from build123d import *

# Parameters (mm, degrees)
SKETCH_1_R          = 21.75
SKETCH_1_R_2        = 14.75
EXTRUDE_1_DEPTH     = 55
CUT_EXTRUDE_START   = -5
SKETCH_2_R          = 18.75
SKETCH_2_R_2        = 14.75
CUT_EXTRUDE_1_DEPTH = 59.016862823
SKETCH_3_R          = 1.25
CUT_EXTRUDE_2_DEPTH = 5


with BuildPart() as part:
    # ｽｹｯﾁ1 → ﾎﾞｽ - 押し出し1 (new body)
    with BuildSketch(Plane(origin=(0, 0, 0), x_dir=(1, 0, 0), z_dir=(0, 1, 0))):
        with Locations(Location((0, 0, 0), (0, 0, 270))):
            Circle(SKETCH_1_R)
        with Locations(Location((0, 0, 0), (0, 0, 270))):
            Circle(SKETCH_1_R_2, mode=Mode.SUBTRACT)
    extrude(amount=EXTRUDE_1_DEPTH)

    # ｽｹｯﾁ2 → ｶｯﾄ - 押し出し1 (cut, through all)
    with BuildSketch(Plane(origin=(0, 55, 0), x_dir=(1, 0, 0), z_dir=(0, 1, 0)).offset(CUT_EXTRUDE_START)):
        with Locations(Location((0, 0, 0), (0, 0, 270))):
            Circle(SKETCH_2_R)
        with Locations(Location((0, 0, 0), (0, 0, 270))):
            Circle(SKETCH_2_R_2, mode=Mode.SUBTRACT)
    extrude(amount=-CUT_EXTRUDE_1_DEPTH, mode=Mode.SUBTRACT)

    # ｽｹｯﾁ3 → ｶｯﾄ - 押し出し2 (cut)
    with BuildSketch(Plane(origin=(0, 55, 0), x_dir=(1, 0, 0), z_dir=(0, 1, 0))):
        with Locations(Location((0, 18.25, 0), (0, 0, 270))):
            Circle(SKETCH_3_R)
        with Locations(Location((18.25, 0, 0), (0, 0, 270))):
            Circle(SKETCH_3_R)
        with Locations(Location((0, -18.25, 0), (0, 0, 270))):
            Circle(SKETCH_3_R)
        with Locations(Location((-18.25, 0, 0), (0, 0, 270))):
            Circle(SKETCH_3_R)
    extrude(amount=-CUT_EXTRUDE_2_DEPTH, mode=Mode.SUBTRACT)


solid = part.part
Geometry check sheet. Reference: the model listing, model coordinates, mm. A direction names the side the tool comes from. Give positions to 0.01 mm unless a question says otherwise; leave off trailing zeros. Order: outer loops, then holes, each group sorted by start corner. A loop starts at its lowest first (then second) coordinate and runs counter-clockwise, first axis right, second up.
1) Cross-section at C-C (x = 10). Record the boundary of the cut face in (y, z), then the cut area to 3 significant figures.
Results are:
outline: (0, -19.31) - (55, -19.31) - (55, -10.84) - (50, -10.84) - (50, -15.86) - (0, -15.86) - close; (0, 15.86) - (50, 15.86) - (50, 10.84) - (55, 10.84) - (55, 19.31) - (0, 19.31) - close
area: 430 mm2
2) Gauge pin test, flat ends, axial feed: pin 1 (10 mm diameter, centred on x = -2.5, y = 13, fed in from +Z); pin 2 (2 mm diameter, centred on x = 0, z = -18.25, fed in from +Y); pin 3 (3 mm diameter, centred on x = -15, y = 7.5, fed in from -Z); pin 4 (2 mm diameter, centred on x = -4.5, y = 8.5, fed in from -Z). Record the tip position at first contact, or that the pin passes through.
Results are:
pin 1: stops at z = 21.75
pin 2: stops at y = 50
pin 3: stops at z = -17.05
pin 4: stops at z = -21.47
3) Cross-section at B-B (z = 0). Record the boundary of the cut face in (x, y).
Results are:
outline: (-21.75, 0) - (-18.75, 0) - (-18.75, 50) - (-19.5, 50) - (-19.5, 55) - (-21.75, 55) - close; (-17, 50) - (-14.75, 50) - (-14.75, 55) - (-17, 55) - close; (14.75, 50) - (17, 50) - (17, 55) - (14.75, 55) - close; (18.75, 0) - (21.75, 0) - (21.75, 55) - (19.5, 55) - (19.5, 50) - (18.75, 50) - close
4) Draft check along X on faces 1 (the flat face through (15, 55, 0)), 2 (the flat face through (-12.4, 50, -8.4)), 3 (the cylindrical face through (21.565, 27.115, -2.831)). Enter one of: released by +X, released by -X, zero draft, split by the parting line, or undercut.
Results are:
face 1: zero draft
face 2: undercut
face 3: split by the parting line
5) Tool access check on faces 4 (the cylindrical face through (-11.41, 25.35, -14.88)), 5 (the cylindrical face through (-19.47, 52.54, -0.27)), 6 (the flat face through (18, 0, 6)). Record the directions out of +Z, -Z, +X, -X, +Y, -Y that give a thin tool (end or side, any length) a straight path to the whole face; none if there is none.
Results are:
face 4: -Y
face 5: +Y
face 6: +Z, -Z, +X, -X, -Y
6) Cross-section at A-A (x = 0). Record the boundary of the cut face in (y, z).
Results are:
outline: (0, -21.75) - (55, -21.75) - (55, -19.5) - (50, -19.5) - (50, -18.75) - (0, -18.75) - close; (0, 18.75) - (50, 18.75) - (50, 19.5) - (55, 19.5) - (55, 21.75) - (0, 21.75) - close; (50, -17) - (55, -17) - (55, -14.75) - (50, -14.75) - close; (50, 14.75) - (55, 14.75) - (55, 17) - (50, 17) - close
7) Material ranges on probe 1 along X at (y, z) = (53.85, 0); probe 2 along Y at (x, z) = (17.5, 5); probe 3 along Z at (x, y) = (18, 51), recorded low to high.
Results are:
probe 1: x = -21.75 to -19.5, -17 to -14.75, 14.75 to 17, 19.5 to 21.75
probe 2: y = 50 to 55
probe 3: z = -12.21 to -1.22, 1.22 to 12.21
8) Cross-section at D-D (z = -6). Record the boundary of the cut face in (x, y), then the cut area to 3 significant figures.
Results are:
outline: (-20.91, 0) - (-17.76, 0) - (-17.76, 50) - (-13.47, 50) - (-13.47, 55) - (-20.91, 55) - close; (13.47, 50) - (17.76, 50) - (17.76, 0) - (20.91, 0) - (20.91, 55) - (13.47, 55) - close
area: 389 mm2
